Can you work these out from the model? Positions are in its coordinate system, mm. Coordinates: 2 decimals unless noted, no trailing zeros. Order: outer loops, then holes, each group sorted by start corner. A loop starts at its lowest first (then second) coordinate and runs counter-clockwise, first axis right, second up. Notation, with made-up numbers: (41.5, 2) -> (45.5, 2) arc R28 ccw to (45.5, 24) -> close; hole circle Ø7 at (-30.5, 40.25). An arc over 180 degrees is marked (long way). Answer in a Markdown table with one row per item. Add a question column.
1. Imagine slicing it at B-B on y = 1.8. State how many separate pieces and enclosed holes the cut face has, plus the area to 3 significant figures.
2. We'd pull the mould along X, two halves only. Please class faces 1 (the face through (0.391, 1.479, -17.317)), 2 (the face through (0, 0, 73)), 3 (the face through (-19.142, 1.479, -23.891)), 4 (the face through (11.696, 1.479, -31.689)): pulls with the +X half, pulls with the -X half, needs draft (parallel to the pull), parting line crosses it, or undercut.
3. If I drill on line 1 along Z through (x, y) = (8, 1.3); line 2 along Z through (x, y) = (6, 1.95); line 3 along X through (y, z) = (1.25, 139.5), over which ranges is the centre line in solid material (lowest first)? Write a range as [from, to].
4. Imagine slicing it at A-A on z = 81. Write out the boundary of the cut face in (x, y).
5. Will these pins go through, and if not, where does the flat tip stop? pin 1 (2.5 mm diameter, centred on x = 6, z = 151.87, fed in from -Y); pin 2 (5 mm diameter, centred on x = 0, z = 139.44, fed in from -Y); pin 3 (1.5 mm diameter, centred on x = 4.5, y = 1, fed in from +Z).
Autodesk Inventor part; units mm, degrees
ref_plane "YZ Plane" through (0, 0, 0) normal (1, 0, 0) x (0, 1, 0)
ref_plane "XZ Plane" through (0, 0, 0) normal (0, 1, 0) x (-1, 0, 0)
ref_plane "XY Plane" through (0, 0, 0) normal (0, 0, 1) x (1, 0, 0)
sketch "Sketch3" plane through (0, 0, 0) normal (0, 1, 0) x (-1, 0, 0)
  line L0 (6.6262, -36.1747) -> (16.6262, -27.3275)
  arc A0 (16.6262, -27.3275) -> (20, -19.8379) centre (10, -19.8379) ccw
  line L1 (20, -19.8379) -> (20, -7.6759)
  arc A1 (20, -7.6759) -> (18, -1.6759) centre (10, -7.6759) ccw
  line L2 (18, -1.6759) -> (14.5, 2.9908)
  arc A2 (12.5, 8.9908) -> (14.5, 2.9908) centre (22.5, 8.9908) ccw
  arc A3 (-14.5, 2.9908) -> (-12.5, 8.9908) centre (-22.5, 8.9908) ccw
  line L3 (-14.5, 2.9908) -> (-18, -1.6759)
  arc A4 (-18, -1.6759) -> (-20, -7.6759) centre (-10, -7.6759) ccw
  line L4 (-20, -7.6759) -> (-20, -19.8379)
  arc A5 (-20, -19.8379) -> (-16.6262, -27.3275) centre (-10, -19.8379) ccw
  line L5 (-16.6262, -27.3275) -> (-6.6262, -36.1747)
  arc A6 (-6.6262, -36.1747) -> (6.6262, -36.1747) centre (0, -28.6852) ccw
  line L6 (-7.8135, -19.9641) -> (-6.7529, -18.9034)
  arc A7 (-4.5608, -21.0955) -> (-6.7529, -18.9034) centre (-5.6569, -19.9994) ccw
  line L7 (-4.5608, -21.0955) -> (-5.6215, -22.1561)
  arc A8 (-7.8135, -19.9641) -> (-5.6215, -22.1561) centre (-6.7175, -21.0601) ccw
  arc A9 (5.6215, -22.1561) -> (7.8135, -19.9641) centre (6.7175, -21.0601) ccw
  line L8 (5.6215, -22.1561) -> (4.5608, -21.0955)
  arc A10 (6.7529, -18.9034) -> (4.5608, -21.0955) centre (5.6569, -19.9994) ccw
  line L9 (6.7529, -18.9034) -> (7.8135, -19.9641)
  arc A11 (-6.7529, -9.7817) -> (-4.5608, -7.5897) centre (-5.6569, -8.6857) ccw
  line L10 (-6.7529, -9.7817) -> (-7.8135, -8.7211)
  arc A12 (-5.6215, -6.5291) -> (-7.8135, -8.7211) centre (-6.7175, -7.6251) ccw
  line L11 (-5.6215, -6.5291) -> (-4.5608, -7.5897)
  arc A13 (7.8135, -8.7211) -> (5.6215, -6.5291) centre (6.7175, -7.6251) ccw
  line L12 (7.8135, -8.7211) -> (6.7529, -9.7817)
  arc A14 (4.5608, -7.5897) -> (6.7529, -9.7817) centre (5.6569, -8.6857) ccw
  line L13 (4.5608, -7.5897) -> (5.6215, -6.5291)
  circle A15 centre (0, -14.3426) radius 3
  line L14 (-12.5, 8.9908) -> (12.5, 8.9908) construction
  arc A16 (12.5, 149.6916) -> (12.2297, 154.0328) centre (-22.5, 149.6916) ccw
  line L15 (12.2297, 154.0328) -> (10, 171.8706)
  line L16 (10, 171.8706) -> (10, 179.8706)
  arc A17 (10, 179.8706) -> (8, 181.8706) centre (8, 179.8706) ccw
  line L17 (8, 181.8706) -> (2, 181.8706)
  arc A18 (2, 181.8706) -> (0, 179.8706) centre (2, 179.8706) ccw
  line L18 (0, 179.8706) -> (0, 173.8706)
  arc A19 (-2, 171.8706) -> (0, 173.8706) centre (-2, 173.8706) ccw
  line L19 (-2, 171.8706) -> (-8.2344, 171.8706)
  arc A20 (-8.2344, 171.8706) -> (-10.219, 170.1187) centre (-8.2344, 169.8706) ccw
  line L20 (-10.219, 170.1187) -> (-12.2297, 154.0328)
  arc A21 (-12.2297, 154.0328) -> (-12.5, 149.6916) centre (22.5, 149.6916) ccw
  circle A22 centre (6, 151.8706) radius 1.5
  circle A23 centre (-6, 151.8706) radius 1.5
  circle A24 centre (0, 139.4442) radius 1.5
  circle A25 centre (0, 160.6574) radius 4
  line L21 (-12.5, 149.6916) -> (12.5, 149.6916) construction
  line L22 (0, -14.3426) -> (0, 160.6574) construction
  line L23 (12.5, 8.9908) -> (12.5, 149.6916)
  line L24 (-12.5, 149.6916) -> (-12.5, 8.9908)
  dimension "d4" = 21.2132
  dimension "d7" = 12
  dimension "d10" = 175
extrude "Extrusion1" add sketch "Sketch3" along normal blind 3
sketch "Sketch4" plane through (0, 3, 0) normal (0, 1, 0) x (1, 0, 0)
  circle A0 centre (0, 14.3426) radius 3 construction
  circle A1 centre (0, 14.3426) radius 88.9 construction
  circle A2 centre (0, -160.6574) radius 4
  point P0 (0, 0)
  dimension "d9" = 177.8
  dimension "d11" = 175
sketch "Sketch5" plane through (0, 3, 0) normal (0, 1, 0) x (1, 0, 0)
  line L0 (-18, 1.6759) -> (-14.5, -2.9908)
  arc A0 (-12.5, -8.9908) -> (-14.5, -2.9908) centre (-22.5, -8.9908) ccw
  line L1 (-12.5, -8.9908) -> (-12.5, -149.6916)
  line L2 (14.5, -2.9908) -> (18, 1.6759)
  arc A1 (14.5, -2.9908) -> (12.5, -8.9908) centre (22.5, -8.9908) ccw
  line L3 (12.5, -149.6916) -> (12.5, -8.9908)
  circle A2 centre (0, 14.3426) radius 3 construction
  circle A3 centre (0, -139.4442) radius 1.5 construction
  line L4 (0, 14.3426) -> (0, -139.4442) construction
  line L5 (7.5, 14.3426) -> (7.5, -139.4442)
  line L6 (-7.5, 14.3426) -> (-7.5, -139.4442)
  arc A4 (14.5, -2.9908) -> (12.5, -8.9908) centre (22.5, -8.9908) ccw
  line L7 (14.5, -2.9908) -> (5.7311, -14.6826)
  arc A5 (-12.5, -8.9908) -> (-14.5, -2.9908) centre (-22.5, -8.9908) ccw
  line L8 (-14.5, -2.9908) -> (-5.817, -14.5681)
  circle A6 centre (0, 14.3426) radius 88.9 construction
  line L9 (7.5, -74.2405) -> (12.5, -80.9071)
  line L10 (-7.5, -74.2405) -> (-12.5, -80.9071)
  point P0 (0, 0)
  point P1 (7.5, -12.3241)
  point P2 (-7.5, -12.3241)
  dimension "d12" = 7.5
  dimension "d13" = 7.5
  dimension "d14" = 143.13
  dimension "d15" = 143.13
  dimension "d16" = 143.13
extrude "Extrusion2" [suppressed]
fillet "Fillet1" [suppressed]
properties part number "Kauri arm long"
Answers follow:
| question | item | result |
|---|---|---|
| 1 | separate pieces | 1 |
| 1 | enclosed holes | 9 |
| 1 | area | 5,510 mm² |
| 2 | face 1 | undercut |
| 2 | face 2 | needs draft |
| 2 | face 3 | pulls with the -X half |
| 2 | face 4 | pulls with the +X half |
| 3 | line 1 | z = [-34.96, -21.93], [-20.19, -8.5], [-6.75, 171.87] |
| 3 | line 2 | z = [-36.69, -22.43], [-18.49, -10.2], [-6.25, 150.37], [153.37, 171.87] |
| 3 | line 3 | x = [-12.5, -1.5], [1.5, 12.5] |
| 4 | outline | (-12.5, 0) -> (12.5, 0) -> (12.5, 3) -> (-12.5, 3) -> close |
| 5 | pin 1 | passes through |
| 5 | pin 2 | stops at y = 0 |
| 5 | pin 3 | stops at z = 171.87 |
